Here's the drawing with two shaded views (mm, measured from the low corner). I have some questions. A direction names the side the tool comes from. Coordinates: 2 decimals unless noted, no trailing zeros. Write each loop counter-clockwise with the first axis right and the second up, starting at its lowest first coordinate (ties: lowest second). Pieces come first, ordered by that corner, then holes. Notation, with made-up numbers: (68.5, 83.25) -> (118.5, 83.25) arc R17 ccw to (118.5, 102.25) -> close; hole circle Ø9 at (12.5, 36). An arc over 180 degrees is marked (long way). Use a Markdown table: item, result. Add a question column.
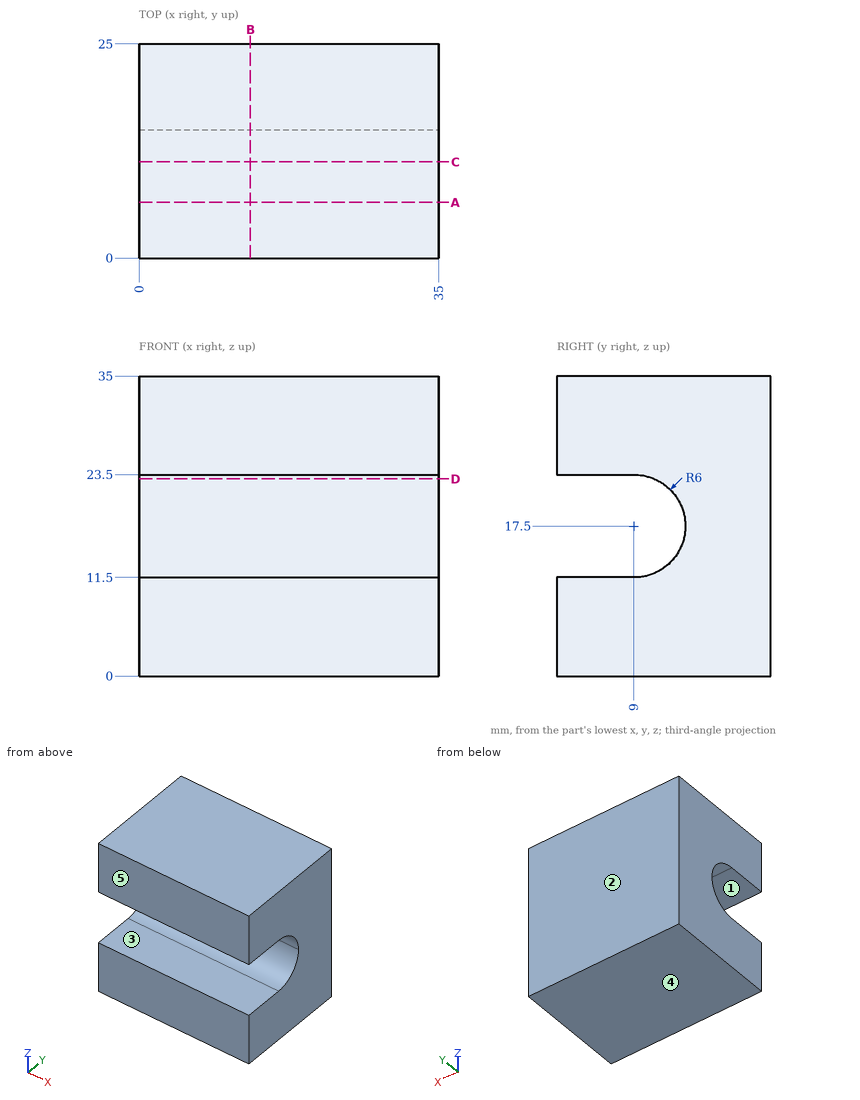
Q1. Suppose I cut it at C-C, the plane y = 11.25. Write out the boundary of the cut face in (x, z), and give its area (3 significant figures).
Q2. Suppose I cut it at D-D, the plane z = 23. Write out the boundary of the cut face in (x, y).
Q3. Please list where these lines run through material, in increasing order: line 1 (Z direction, x = 23.5, y = 5.25); line 2 (Y direction, x = 18, z = 16); line 3 (Y direction, x = 26, z = 17).
Q4. Suppose I cut it at A-A, the plane y = 6.5. Write out the boundary of the cut face in (x, z).
Q5. Will these pins go through, and if not, where does the flat tip stop? pin 1 (8 mm diameter, centred on y = 10.5, z = 17.5, fed in from +X); pin 2 (3 mm diameter, centred on x = 28.5, z = 23, fed in from -Y).
Q6. Suppose I cut it at B-B, the plane x = 13. Write out the boundary of the cut face in (y, z).
Q7. Thinking about a two-plate mould opening in Z: for the marked faces 3, 4 and 5, which applies, released by +Z, released by -Z, zero draft, split by the parting line, or undercut?
Q8. Which directions (+Z, -Z, +X, -X, +Y, -Y) give clear straight access to the entire face, cutting with the end or side of a thin tool? Please do the marked faces 1 and 2.
Answer key:
| question | item | result |
|---|---|---|
| 1 | outline | (0, 0) -> (35, 0) -> (35, 11.94) -> (0, 11.94) -> close; (0, 23.06) -> (35, 23.06) -> (35, 35) -> (0, 35) -> close |
| 1 | area | 836 mm^2 |
| 2 | outline | (0, 11.4) -> (35, 11.4) -> (35, 25) -> (0, 25) -> close |
| 3 | line 1 | z = 0 to 11.5, 23.5 to 35 |
| 3 | line 2 | y = 14.81 to 25 |
| 3 | line 3 | y = 14.98 to 25 |
| 4 | outline | (0, 0) -> (35, 0) -> (35, 11.5) -> (0, 11.5) -> close; (0, 23.5) -> (35, 23.5) -> (35, 35) -> (0, 35) -> close |
| 5 | pin 1 | passes through |
| 5 | pin 2 | stops at y = 0 |
| 6 | outline | (0, 0) -> (25, 0) -> (25, 35) -> (0, 35) -> (0, 23.5) -> (9, 23.5) arc R6 cw to (9, 11.5) -> (0, 11.5) -> close |
| 7 | face 3 | undercut |
| 7 | face 4 | released by -Z |
| 7 | face 5 | zero draft |
| 8 | face 1 | +X, -X, -Y |
| 8 | face 2 | +Z, -Z, +X, -X, +Y |
